For this review, take the finished solid that the model builds, in its own axes (mm). Face numbers are marked on the shaded views. A direction names the side the tool comes from. Round coordinates to 2 decimals unless told otherwise and drop trailing zeros. Order: outer loops, then holes, each group sorted by start corner. A loop starts at its lowest first (then second) coordinate and runs counter-clockwise, first axis right, second up. Notation, with made-up numbers: (33, -13.5) -> (56, -13.5) arc R22 cw to (56, 3.5) -> close; hole circle Ø6 at (7.25, 63.5). An arc over 180 degrees is marked (long way). Use a Markdown table: item, result. Add a question column.
1) Consider section B-B (z = 35). State the section outline as (x, y) points, plus the area to 3 significant figures.
2) Machinability: for the marked faces 1, 2, 3, 4 and 5, which of the approach directions +Z, -Z, +X, -X, +Y, -Y give a long, thin tool a straight path to every point of the face, cutting with its end or side? Answer none if there is none.
3) Consider section A-A (y = 52). State the section outline as (x, z) points.
4) Consider section C-C (x = 35). State the section outline as (y, z) points, plus the area to 3 significant figures.
5) Draft analysis for pull direction Y (two halves, no side actions). For the marked faces 6, 7, 8 and 9, state which applies: pulls with the +Y half, pulls with the -Y half, needs draft (parallel to the pull), parting line crosses it, or undercut.
6) Consider section D-D (z = 6.5). State the section outline as (x, y) points.
7) Wall thickness on line 1 along Z through (x, y) = (0, -4.35); line 2 along Z through (x, y) = (8, 59); line 3 along Y through (x, z) = (-15, -24.5): over which ranges is each line inside the solid? List them lowest first. Write a range as [from, to].
8) Clearance check with flat-ended pins moving along their axes: P1, Ø1.9, axis at x = -35.5, y = -1.5, coming from the -Z side; P2, Ø0.7, axis at x = 35.5, y = -1.5, coming from the +Z side; P3, Ø2.5, axis at x = -34.5, y = -1.5, coming from the +Z side; P4, Ø2, axis at x = 35, z = 0, coming from the +Y side. State where each tip first meets the part, or that it passes through.
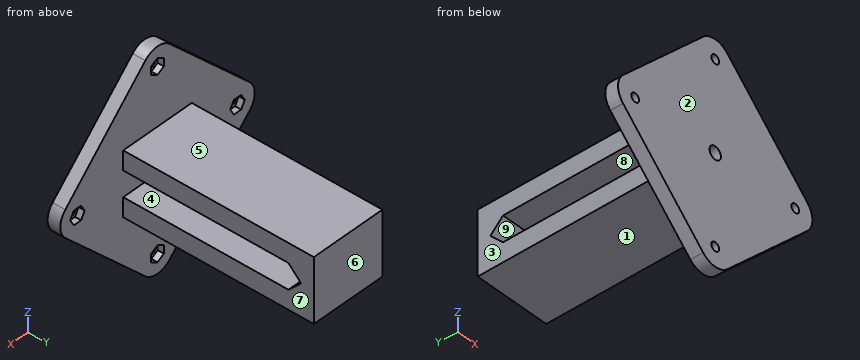
Autodesk Inventor part; units mm, degrees
ref_plane "YZ Plane" through (0, 0, 0) normal (1, 0, 0) x (0, 1, 0)
ref_plane "XZ Plane" through (0, 0, 0) normal (0, 1, 0) x (-1, 0, 0)
ref_plane "XY Plane" through (0, 0, 0) normal (0, 0, 1) x (1, 0, 0)
sketch "Sketch1" plane through (0, 0, 0) normal (0, 1, 0) x (-1, 0, 0)
  circle A0 centre (0, 0) radius 17.5 construction
  line L0 (0, 35) -> (0, -35) construction
  line L1 (35, 0) -> (-35, 0) construction
  dimension "d0" = 35
  dimension "d1" = 70
  dimension "d2" = 70
sketch "Sketch2" plane through (0, 0, 0) normal (0, 1, 0) x (-1, 0, 0)
  circle A0 centre (0, 0) radius 17.5 construction
  line L0 (0, 35) -> (0, -35) construction
  line L1 (35, 0) -> (-35, 0) construction
  circle A1 centre (35, 0) radius 7.5
  circle A2 centre (0, 35) radius 7.5
  circle A3 centre (-35, 0) radius 7.5
  circle A4 centre (0, -35) radius 7.5
  line L2 (5.3033, 40.3033) -> (40.3033, 5.3033)
  line L3 (-40.3033, 5.3033) -> (-5.3033, 40.3033)
  line L4 (-5.3033, -40.3033) -> (-40.3033, -5.3033)
  line L5 (40.3033, -5.3033) -> (5.3033, -40.3033)
  circle A5 centre (0, 0) radius 2.5
  point P0 (5.3033, -40.3033)
  point P1 (-40.3033, -5.3033)
  dimension "d3" = 15
  dimension "d6" = 360
  dimension "d10" = 360
  dimension "d14" = 5
extrude "Extrusion1" add sketch "Sketch2" against normal blind 5
hole "Hole1" at (0, 0, -35) at (0, 0, 35) at (-35, 0, 0) at (35, 0, 0) direction (0, -1, 0) diameter 3.4 end through all
sketch "Sketch3" plane through (0, 0, 0) normal (0, 1, 0) x (1, 0, 0)
  line L0 (15, -12.5) -> (-15, -12.5)
  line L1 (-15, -12.5) -> (-15, 12.5)
  line L2 (-15, 12.5) -> (15, 12.5)
  line L3 (15, 12.5) -> (15, -12.5)
  circle A0 centre (0, 0) radius 2.5
  line L4 (15, -12.5) -> (-15, 12.5) construction
  line L5 (-15, -12.5) -> (15, 12.5) construction
  line L6 (15, -5) -> (-15, -5)
  line L7 (-15, -5) -> (-15, 5)
  line L8 (-15, 5) -> (15, 5)
  line L9 (15, 5) -> (15, -5)
  line L10 (15, -5) -> (-15, 5) construction
  line L11 (-15, -5) -> (15, 5) construction
  point P0 (15, -5)
  dimension "d22" = 30
  dimension "d23" = 25
  dimension "d24" = 10
extrude "Extrusion2" add sketch "Sketch3" along normal blind 70 contours L0 L1 L6 L3 | L8 L1 L2 L3
sketch "Sketch4" plane through (0, 70, 0) normal (0, 1, 0) x (1, 0, 0)
  line L0 (-15, 12.5) -> (15, 12.5)
  line L1 (15, 12.5) -> (15, -12.5)
  line L2 (15, -12.5) -> (-15, -12.5)
  line L3 (-15, -12.5) -> (-15, 12.5)
  point P0 (0, 0)
extrude "Extrusion3" add sketch "Sketch4" along normal blind 5
sketch "Sketch5" plane through (0, 0, 0) normal (0, 1, 0) x (1, 0, 0)
  line L0 (15, -12.5) -> (-15, -12.5)
  line L1 (-15, -12.5) -> (-15, -5)
  line L2 (-15, -5) -> (15, -5)
  line L3 (15, -5) -> (15, -12.5)
  line L4 (-15, 12.5) -> (15, 12.5)
  line L5 (15, 12.5) -> (15, 5)
  line L6 (15, 5) -> (-15, 5)
  line L7 (-15, 5) -> (-15, 12.5)
  circle A0 centre (35, 0) radius 1.7
  circle A1 centre (-35, 0) radius 1.7
  circle A2 centre (0, -35) radius 1.7
  circle A3 centre (0, 35) radius 1.7
  arc A4 (-40.3033, 5.3033) -> (-40.3033, -5.3033) centre (-35, 0) ccw
  line L8 (-40.3033, -5.3033) -> (-5.3033, -40.3033)
  arc A5 (-5.3033, -40.3033) -> (5.3033, -40.3033) centre (0, -35) ccw
  line L9 (5.3033, -40.3033) -> (40.3033, -5.3033)
  arc A6 (40.3033, -5.3033) -> (40.3033, 5.3033) centre (35, 0) ccw
  line L10 (40.3033, 5.3033) -> (5.3033, 40.3033)
  arc A7 (5.3033, 40.3033) -> (-5.3033, 40.3033) centre (0, 35) ccw
  line L11 (-5.3033, 40.3033) -> (-40.3033, 5.3033)
  circle A8 centre (0, 0) radius 2.5
  circle A9 centre (-35, 0) radius 2.75 construction
  line L12 (-33.4123, 2.75) -> (-31.8246, 0)
  line L13 (-31.8246, 0) -> (-33.4123, -2.75)
  line L14 (-33.4123, -2.75) -> (-36.5877, -2.75)
  line L15 (-36.5877, -2.75) -> (-38.1754, 0)
  line L16 (-38.1754, 0) -> (-36.5877, 2.75)
  line L17 (-36.5877, 2.75) -> (-33.4123, 2.75)
  line L18 (-2.75, -33.4123) -> (0, -31.8246)
  line L19 (0, -31.8246) -> (2.75, -33.4123)
  circle A10 centre (0, -35) radius 2.75 construction
  line L20 (0, -38.1754) -> (-2.75, -36.5877)
  line L21 (2.75, -36.5877) -> (0, -38.1754)
  line L22 (2.75, -33.4123) -> (2.75, -36.5877)
  line L23 (-2.75, -36.5877) -> (-2.75, -33.4123)
  line L24 (33.4123, -2.75) -> (31.8246, 0)
  line L25 (31.8246, 0) -> (33.4123, 2.75)
  circle A11 centre (35, 0) radius 2.75 construction
  line L26 (38.1754, 0) -> (36.5877, -2.75)
  line L27 (36.5877, 2.75) -> (38.1754, 0)
  line L28 (33.4123, 2.75) -> (36.5877, 2.75)
  line L29 (36.5877, -2.75) -> (33.4123, -2.75)
  line L30 (2.75, 33.4123) -> (0, 31.8246)
  line L31 (0, 31.8246) -> (-2.75, 33.4123)
  circle A12 centre (0, 35) radius 2.75 construction
  line L32 (0, 38.1754) -> (2.75, 36.5877)
  line L33 (-2.75, 36.5877) -> (0, 38.1754)
  line L34 (-2.75, 33.4123) -> (-2.75, 36.5877)
  line L35 (2.75, 36.5877) -> (2.75, 33.4123)
  point P0 (-35, 2.75)
  point P1 (-2.75, -35)
  point P2 (35, -2.75)
  point P3 (2.75, 35)
  dimension "d29" = 5.5
  dimension "d32" = 360
extrude "Extrusion4" cut sketch "Sketch5" against normal blind 2.4 contours A0 | A1 | A2 | L12 L13 L14 L15 L16 L17 | L18 L19 L22 L21 L20 L23 | L24 L25 L28 L27 L26 L29 | L30 L31 L34 L33 L32 L35
chamfer "Chamfer1" distance 5 angle 45 2 edges at (0, 70, -5) (0, 70, 5)
properties part number "turning prevention"
Results list:
| question | item | result |
|---|---|---|
| 1 | outline | (-10.61, -5) -> (-1.7, -5) -> (-1.7, -2.4) -> (-2.75, -2.4) -> (-2.75, 0) -> (-10.61, 0) -> close; (1.7, -5) -> (10.61, -5) -> (10.61, 0) -> (2.75, 0) -> (2.75, -2.4) -> (1.7, -2.4) -> close |
| 1 | area | 84.0 mm2 |
| 2 | face 1 | -Z, +X, -X, +Y |
| 2 | face 2 | +Z, -Z, +X, -X, -Y |
| 2 | face 3 | +Z, -Z, -X, +Y |
| 2 | face 4 | +X, -X |
| 2 | face 5 | +Z, +X, -X, +Y |
| 3 | outline | (-15, -12.5) -> (15, -12.5) -> (15, -5) -> (-15, -5) -> close; (-15, 5) -> (15, 5) -> (15, 12.5) -> (-15, 12.5) -> close |
| 4 | outline | (-5, -10.61) -> (0, -10.61) -> (0, -2.75) -> (-2.4, -2.75) -> (-2.4, -1.7) -> (-5, -1.7) -> close; (-5, 1.7) -> (-2.4, 1.7) -> (-2.4, 2.75) -> (0, 2.75) -> (0, 10.61) -> (-5, 10.61) -> close |
| 4 | area | 84.0 mm2 |
| 5 | face 6 | pulls with the +Y half |
| 5 | face 7 | needs draft |
| 5 | face 8 | undercut |
| 5 | face 9 | undercut |
| 6 | outline | (-39.11, -5) -> (39.11, -5) -> (39.11, 0) -> (15, 0) -> (15, 75) -> (-15, 75) -> (-15, 0) -> (-39.11, 0) -> close |
| 7 | line 1 | [-42.5, -36.7], [-33.3, -2.5], [2.5, 33.3], [36.7, 42.5] |
| 7 | line 2 | [-12.5, -5], [5, 12.5] |
| 7 | line 3 | [-5, 0] |
| 8 | P1 | z = -11.06 |
| 8 | P2 | z = 10.46 |
| 8 | P3 | z = 12.36 |
| 8 | P4 | through |
